from build123d import *

# Parameters (mm, degrees)
F1_DEPTH = 2


with BuildPart() as f1:
    # F0 (on Top) → F1 (new body, symmetric)
    with BuildSketch(Plane.XY):
        Polygon((0, 62), (0, 0), (0, -62), (45, -62), (45, -40), (115, -40), (115, -62), (245, -98.081973), (245, -40), (315, -40), (315, -98.081973), (359, -62), (359, 0), (359, 62), (315, 98.081973), (315, 40), (245, 40), (245, 98.081973), (115, 62), (115, 40), (45, 40), (45, 62), align=None)
    extrude(amount=F1_DEPTH, both=True)


solid = f1.part
Verification items for the finished model (mm, model axes). Give positions to 0.01 mm unless a question says otherwise; leave off trailing zeros. Order: outer loops, then holes, each group sorted by start corner. A loop starts at its lowest first (then second) coordinate and runs counter-clockwise, first axis right, second up. Notation, with made-up numbers: M 15,-16.5 L 19,-16.5 A20 ccw 19,-2.5 Z; hole C 39.25,55 d10. An arc over 180 degrees is marked long. Answer as a JSON object with one key per item and string values. Group by question number.
1) Cross-section at B-B (y = -85). Enter the section's corners in (x, z), then the cut area to 3 significant figures.
2) Cross-section at D-D (x = 69). Enter the section's corners in (y, z), then the cut area to 3 significant figures.
3) Cross-section at A-A (y = 44). Enter the section's corners in (x, z).
4) Cross-section at C-C (z = -0.1). Enter the section's corners in (x, y), then the cut area to 3 significant figures.
5) Scan lines: line 1 along X through (y, z) = (-43.5, -0.2); line 2 along Y through (x, z) = (106.5, 1.2); line 3 along Y through (x, z) = (15, -1.75). Record each from-to range of solid material in increasing order. Write a range as [from, to].
6) Depth check by flat-ended pin: pin 1 Ø1.2 at (y, z) = (-82, 0.5) entering from +X; pin 2 Ø1.2 at (x, z) = (82, -0.5) entering from -Y; pin 3 Ø1.2 at (x, z) = (19.5, -0.5) entering from -Y. Enter the tip coordinate at first touch or a pass-through.
Result sheet:
{
 "1": {"outline": "M 197.87,-2 L 245,-2 L 245,2 L 197.87,2 Z; M 315,-2 L 330.95,-2 L 330.95,2 L 315,2 Z", "area": "252 mm2"},
 "2": {"outline": "M -40,-2 L 40,-2 L 40,2 L -40,2 Z", "area": "320 mm2"},
 "3": {"outline": "M 0,-2 L 45,-2 L 45,2 L 0,2 Z; M 115,-2 L 245,-2 L 245,2 L 115,2 Z; M 315,-2 L 359,-2 L 359,2 L 315,2 Z"},
 "4": {"outline": "M 0,-62 L 45,-62 L 45,-40 L 115,-40 L 115,-62 L 245,-98.08 L 245,-40 L 315,-40 L 315,-98.08 L 359,-62 L 359,62 L 315,98.08 L 315,40 L 245,40 L 245,98.08 L 115,62 L 115,40 L 45,40 L 45,62 L 0,62 Z", "area": "44,600 mm2"},
 "5": {"line 1": "x = [0, 45], [115, 245], [315, 359]", "line 2": "y = [-40, 40]", "line 3": "y = [-62, 62]"},
 "6": {"pin 1": "stops at x = 335.34", "pin 2": "stops at y = -40", "pin 3": "stops at y = -62"}
}
